Here's how the part is built. I have some questions about the finished solid (model axes, mm). A direction names the side the tool comes from. Round coordinates to 2 decimals unless told otherwise and drop trailing zeros. Order: outer loops, then holes, each group sorted by start corner. A loop starts at its lowest first (then second) coordinate and runs counter-clockwise, first axis right, second up. Notation, with made-up numbers: (55, -26) - (70, -26) arc R20 cw to (70, 6) - close; hole circle Ø9 at (63, 76.25). An arc over 180 degrees is marked (long way). Answer as a JSON object with one key per item and string values.
```python
from build123d import *

# Parameters (mm, degrees)
F1_DEPTH      = 102.108
F2_R          = 28.09345
F3_DEPTH      = 101.6
F3_FACE_R     = 28.09345
F4_DEPTH      = 101.6
F5_R          = 27.192534
F6_DEPTH      = 101.6
F7_R          = 28.729742
F8_DEPTH      = 50.8
F8_DEPTH_BACK = 152.4


with BuildPart() as f1:
    # F0 (on Front) → F1 (new body)
    with BuildSketch(Plane.XZ):
        Polygon((0, 102.652691), (0, 0), (99.562824, 0), (102.996022, 0), (105.399251, 36.73524), (105.399251, 48.408125), (105.399251, 63.514203), (105.399251, 102.652691), align=None)
    extrude(amount=F1_DEPTH)

    # F2 (on face) → F3 (cut)
    with BuildSketch(Plane.XY.offset(102.652691)):
        with Locations((50.061982, -50.997104)):
            Circle(F2_R)
    extrude(amount=-F3_DEPTH, mode=Mode.SUBTRACT)

    # F3_face (on face) → F4 (cut)
    with BuildSketch(Plane(origin=(50.061982, -50.997104, 1.052691), x_dir=(1, 0, 0), z_dir=(0, 0, 1))):
        Circle(F3_FACE_R)
    extrude(amount=-F4_DEPTH, mode=Mode.SUBTRACT)

    # F5 (on face) → F6 (cut)
    with BuildSketch(Plane.XZ.offset(102.108)):
        with Locations((48.267499, 53.63135)):
            Circle(F5_R)
    extrude(amount=-F6_DEPTH, mode=Mode.SUBTRACT)

    # F7 (on Front) → F8 (join, two sides)
    with BuildSketch(Plane.XZ) as f8_sk:
        Circle(F7_R)
    extrude(amount=F8_DEPTH)
    extrude(f8_sk.sketch, amount=-F8_DEPTH_BACK)


solid = f1.part
```
1. For faces 4 (the face through (0, 152.4, 0)), 5 (the face through (74, -73, 0)), 6 (the face through (52, 0, 52)), 7 (the face through (48, -0.508, 54)), 8 (the face through (77, -39, 102.653)), which set-ups out of +Z, -Z, +X, -X, +Y, -Y let a thin tool reach every point of the face, with its end or its side?
Responses:
{"face 4": "+Z, -Z, +X, -X, +Y", "face 5": "-Z, +X, -Y", "face 6": "+Z, +X, +Y", "face 7": "-Y", "face 8": "+Z, +X, -X, +Y, -Y"}
2. Imagine slicing it at A-A (x = 59). List the corners of the cut face in (y, z) for me, plus the area to 3 significant figures.
Responses:
{"outline": "(-102.11, 0) - (-77.63, 0) - (-77.63, 28.65) - (-102.11, 28.65) - close; (-102.11, 78.62) - (-77.63, 78.62) - (-77.63, 102.65) - (-102.11, 102.65) - close; (-24.36, 0) - (0, 0) - (0, 102.65) - (-24.36, 102.65) - (-24.36, 78.62) - (-0.51, 78.62) - (-0.51, 28.65) - (-24.36, 28.65) - close", "area": "2,600 mm2"}
3. For P1, Ø1, axis at x = 74, y = -26, coming from the -Z side; P2, Ø3, axis at x = 3, y = 26.5, coming from the -Z side; P3, Ø12, axis at x = -10.5, z = 70, coming from the -Y side; P4, Ø12, axis at y = -28, z = -11, coming from the -X side, each with a flat end and sliding along its axis, tell me the tip position at first contact or that it passes through.
Responses:
{"P1": "z = 0", "P2": "z = -28.69", "P3": "through", "P4": "x = -28.29"}
4. Imagine slicing it at C-C (y = 99). List the corners of the cut face in (x, z) for me.
Responses:
{"outline": "circle Ø57.46 at (0, 0)"}
5. If I drill on L1, parallel to X at y = -51.5, z = 91; L2, parallel to Y at x = 98, z = 92; L3, parallel to Y at x = 29, z = 34.5, over which ranges is the centre line in solid material (lowest first)? Write a range as [from, to].
Responses:
{"L1": "[0, 21.97], [78.15, 105.4]", "L2": "[-102.11, 0]", "L3": "[-0.51, 0]"}
6. Imagine slicing it at D-D (z = 66). List the corners of the cut face in (x, y) for me, plus the area to 3 significant figures.
Responses:
{"outline": "(0, -102.11) - (24.05, -102.11) - (24.05, -61.61) arc R28.09 cw to (24.05, -40.38) - (24.05, -0.51) - (72.48, -0.51) - (72.48, -34.07) arc R28.09 cw to (72.48, -67.92) - (72.48, -102.11) - (105.4, -102.11) - (105.4, 0) - (0, 0) - close", "area": "5,680 mm2"}
7. Thinking about a two-plate mould opening in Z: for faces 1 (the face through (21.1, -52, 54.8)), 2 (the face through (104.18, -50.34, 18.11)), 3 (the face through (105.399, -50, 69)), which applies, pulls with the +Z half, pulls with the -Z half, needs draft (parallel to the pull), parting line crosses it, or undercut?
Responses:
{"face 1": "undercut", "face 2": "pulls with the -Z half", "face 3": "needs draft"}
8. Imagine slicing it at B-B (z = 13). List the corners of the cut face in (x, y) for me, plus the area to 3 significant figures.
Responses:
{"outline": "(-25.62, -50.8) - (0, -50.8) - (0, -102.11) - (103.85, -102.11) - (103.85, 0) - (25.62, 0) - (25.62, 152.4) - (-25.62, 152.4) - close; hole (21.97, -50.8) arc R28.09 ccw (long way) to (25.62, -37.15) - (25.62, -50.8) - close", "area": "17,300 mm2"}
